CAD build for the part. Positions are in the model's coordinates, mm. A direction names the side the tool comes from. Give positions to 0.01 mm unless a question says otherwise; leave off trailing zeros. Loops run counter-clockwise (first coordinate to the right, second up) from the corner with the lowest first, then second, coordinate; pieces in that order, holes last.
```python
from build123d import *

# Parameters (mm, degrees)
F0_R     = 11.05
F1_DEPTH = 9.2
F2_R     = 11.05
F2_R_2   = 10
F3_DEPTH = 2
F4_R     = 2
F6_DEPTH = 25
F7_SIZE  = 1
F8_SIZE  = 1


with BuildPart() as f1:
    # F0 (on Front) → F1 (new body)
    with BuildSketch(Plane.XZ):
        with BuildLine():
            Line((-10.8594483096, 14.3268800737), (-2.4829795671, 13.8288579597))
            ThreePointArc((-2.4829795671, 13.8288579597), (-12.1676569232, 7.025), (-13.217632082, -4.7641055977))
            Line((-13.217632082, -4.7641055977), (-17.8371662556, 2.2411180703))
            ThreePointArc((-17.8371662556, 2.2411180703), (-34.6870755728, -20.0265924193), (-6.977717946, -16.5679981441))
            Line((-6.977717946, -16.5679981441), (-10.7346525149, -9.064752362))
            ThreePointArc((-10.7346525149, -9.064752362), (0, -14.05), (10.7346525149, -9.064752362))
            Line((10.7346525149, -9.064752362), (6.977717946, -16.5679981441))
            ThreePointArc((6.977717946, -16.5679981441), (34.6870755728, -20.0265924193), (17.8371662556, 2.2411180703))
            Line((17.8371662556, 2.2411180703), (13.217632082, -4.7641055977))
            ThreePointArc((13.217632082, -4.7641055977), (12.1676569232, 7.025), (2.4829795671, 13.8288579597))
            Line((2.4829795671, 13.8288579597), (10.8594483096, 14.3268800737))
            ThreePointArc((10.8594483096, 14.3268800737), (0, 40.0531848387), (-10.8594483096, 14.3268800737))
        make_face()
        with Locations((-21.5623582929, -12.4490333648)):
            Circle(F0_R, mode=Mode.SUBTRACT)
        with Locations((21.5623582929, -12.4490333648)):
            Circle(F0_R, mode=Mode.SUBTRACT)
        Circle(F0_R, mode=Mode.SUBTRACT)
        with Locations((0, 24.8980667296)):
            Circle(F0_R, mode=Mode.SUBTRACT)
    extrude(amount=F1_DEPTH)

    # F2 (on face) → F3 (join)
    with BuildSketch(Plane.XZ.offset(9.2)):
        with Locations((0, 24.8980667296)):
            Circle(F2_R)
        with Locations((0, 24.8980667296)):
            Circle(F2_R_2, mode=Mode.SUBTRACT)
        with Locations((-21.5623582929, -12.4490333648)):
            Circle(F2_R)
        with Locations((-21.5623582929, -12.4490333648)):
            Circle(F2_R_2, mode=Mode.SUBTRACT)
        with Locations((21.5623582929, -12.4490333648)):
            Circle(F2_R)
        with Locations((21.5623582929, -12.4490333648)):
            Circle(F2_R_2, mode=Mode.SUBTRACT)
        Circle(F2_R)
        Circle(F2_R_2, mode=Mode.SUBTRACT)
    extrude(amount=-F3_DEPTH)

    # F4
    f4_edges = [f1.edges().sort_by_distance(p)[0] for p in [
        (2.48298, -4.6, 13.828858),
        (-2.48298, -4.6, 13.828858),
        (-13.217632, -4.6, -4.764106),
        (-10.734653, -4.6, -9.064752),
        (10.734653, -4.6, -9.064752),
        (13.217632, -4.6, -4.764106),
    ]]
    fillet(f4_edges, radius=F4_R)

    # F5 (on face) → F6 (cut)
    with BuildSketch(Plane.XZ.offset(9.2)):
        with BuildLine():
            Line((0, 18.9108662307), (1.7659365324, 21.1738422452))
            ThreePointArc((1.7659365324, 21.1738422452), (0, 24.9152206672), (-1.7659365324, 21.1738422452))
            Line((-1.7659365324, 21.1738422452), (0, 18.9108662307))
        make_face()
        with BuildLine():
            Line((-16.3772905634, -9.4554331154), (-19.2200535463, -9.057575224))
            ThreePointArc((-19.2200535463, -9.057575224), (-21.5772140387, -12.4576103336), (-17.4541170138, -12.1162670212))
            Line((-17.4541170138, -12.1162670212), (-16.3772905634, -9.4554331154))
        make_face()
        with BuildLine():
            Line((16.3772905634, -9.4554331154), (17.4541170138, -12.1162670212))
            ThreePointArc((17.4541170138, -12.1162670212), (21.5772140387, -12.4576103336), (19.2200535463, -9.057575224))
            Line((19.2200535463, -9.057575224), (16.3772905634, -9.4554331154))
        make_face()
    extrude(amount=-F6_DEPTH, mode=Mode.SUBTRACT)

    # F7
    f7_edges = [f1.edges().sort_by_distance(p)[0] for p in [
        (10.530932, 0, 14.307348),
        (8.422362, 0, 12.919623),
        (0, 0, 40.053185),
        (12.167657, 0, 7.025),
        (-10.530932, 0, 14.307348),
        (15.399903, 0, 0.834168),
        (-8.422362, 0, 12.919623),
        (17.655993, 0, 1.96638),
        (-12.167657, 0, 7.025),
        (34.687076, 0, -20.026592),
        (-15.399903, 0, 0.834168),
        (7.125061, 0, -16.273728),
        (-17.655993, 0, 1.96638),
        (6.977541, 0, -13.753791),
        (-34.687076, 0, -20.026592),
        (0, 0, -14.05),
        (-7.125061, 0, -16.273728),
        (-6.977541, 0, -13.753791),
        (-32.612358, 0, -12.449033),
        (10.512358, 0, -12.449033),
        (-11.05, 0, 0),
        (-11.05, 0, 24.898067),
    ]]
    chamfer(f7_edges, length=F7_SIZE)

    # F8#2 (call 1 of 5: OpenCascade refuses the feature's edges together)
    f8_2_edges = [f1.edges().sort_by_distance(p)[0] for p in [
        (-31.562358, -9.2, -12.449033),
    ]]
    chamfer(f8_2_edges, length=F8_SIZE)

    # F8#3 (call 2 of 5)
    f8_3_edges = [f1.edges().sort_by_distance(p)[0] for p in [
        (11.562358, -9.2, -12.449033),
    ]]
    chamfer(f8_3_edges, length=F8_SIZE)

    # F8#4 (call 3 of 5)
    f8_4_edges = [f1.edges().sort_by_distance(p)[0] for p in [
        (-10, -9.2, 0),
    ]]
    chamfer(f8_4_edges, length=F8_SIZE)

    # F8#5 (call 4 of 5)
    f8_5_edges = [f1.edges().sort_by_distance(p)[0] for p in [
        (-10, -9.2, 24.898067),
    ]]
    chamfer(f8_5_edges, length=F8_SIZE)

    # F8 (call 5 of 5)
    f8_edges = [f1.edges().sort_by_distance(p)[0] for p in [
        (10.530932, -9.2, 14.307348),
        (8.422362, -9.2, 12.919623),
        (0, -9.2, 40.053185),
        (12.167657, -9.2, 7.025),
        (-10.530932, -9.2, 14.307348),
        (15.399903, -9.2, 0.834168),
        (-8.422362, -9.2, 12.919623),
        (17.655993, -9.2, 1.96638),
        (-12.167657, -9.2, 7.025),
        (34.687076, -9.2, -20.026592),
        (-15.399903, -9.2, 0.834168),
        (7.125061, -9.2, -16.273728),
        (-17.655993, -9.2, 1.96638),
        (6.977541, -9.2, -13.753791),
        (-34.687076, -9.2, -20.026592),
        (0, -9.2, -14.05),
        (-7.125061, -9.2, -16.273728),
        (-6.977541, -9.2, -13.753791),
    ]]
    chamfer(f8_edges, length=F8_SIZE)


solid = f1.part
```
1. Saw through at A-A, the plane x = 0. Count the separate pieces of the cut face and the enclosed holes in it, and give its area (3 significant figures).
Responses:
separate pieces: 3
enclosed holes: 0
area: 93.5 mm2
2. Tool access for faces 3 (the face through (13, -7.2, -18)), 4 (the face through (15.37, -4.65, 0.84)), 5 (the face through (-34.2, -9.03, -19.2)): list every direction of +Z, -Z, +X, -X, +Y, -Y with a clear straight run to the whole face (end or side of a thin tool).
Responses:
face 3: +Y
face 4: +Y, -Y
face 5: -Y
3. Saw through at B-B, the plane y = -3.75. List the corners of the cut face in (x, z) (3 decimals).
Responses:
outline: (-17.837, 2.241) arc R15.155 ccw (long way) to (-6.978, -16.568) - (-7.272, -15.979) arc R2 cw to (-4.801, -13.204) arc R14.05 ccw to (4.801, -13.204) arc R2 cw to (7.272, -15.979) - (6.978, -16.568) arc R15.155 ccw (long way) to (17.837, 2.241) - (17.475, 1.692) arc R2 cw to (13.836, 2.445) arc R14.05 ccw to (9.035, 10.76) arc R2 cw to (10.202, 14.288) - (10.859, 14.327) arc R15.155 ccw (long way) to (-10.859, 14.327) - (-10.202, 14.288) arc R2 cw to (-9.035, 10.76) arc R14.05 ccw to (-13.836, 2.445) arc R2 cw to (-17.475, 1.692) - close; hole circle Ø22.1 at (-21.562, -12.449); hole circle Ø22.1 at (0, 0); hole circle Ø22.1 at (0, 24.898); hole circle Ø22.1 at (21.562, -12.449)
4. Drop flat-ended pins along their axis: pin 1 (5 mm diameter, centred on x = -15, y = -5, fed in from -Z); pin 2 (3 mm diameter, centred on x = -5, y = -7, fed in from +Z); pin 3 (2 mm diameter, centred on x = -11.5, y = -8, fed in from -Z); pin 4 (17.5 mm diameter, centred on x = -23.5, z = -8, fed in from +Y). Give the stop position or say it passes through.
Responses:
pin 1: stops at z = -27.05
pin 2: stops at z = 39.64
pin 3: stops at z = -24.6
pin 4: stops at y = 0
5. Probe line 1 along X through (y, z) = (-4.5, -13); line 2 along Z through (x, y) = (8.5, -4); line 3 along X through (y, z) = (-2, -17.5). List the from-to ranges inside material, lowest first.
Responses:
line 1: x = -36.71 to -32.6, -10.53 to 10.53, 32.6 to 36.71
line 2: z = -20.13 to -7.06, 7.06 to 11.46, 13.12 to 17.84, 31.96 to 37.45
line 3: x = -35.85 to -31.39, -11.73 to -7.27, 7.27 to 11.73, 31.39 to 35.85
6. Pull direction X, two halves, no side cores. Call faces 1 (the face through (-2.395, -4.057, -10.787)), 2 (the face through (8.433, -4.65, 12.951)): released by +X, released by -X, zero draft, split by the parting line, or undercut.
Responses:
face 1: undercut
face 2: released by +X
